Design review of the part built by this model. Coordinates are the model's own, in mm. A direction names the side the tool comes from. Round coordinates to 2 decimals unless told otherwise and drop trailing zeros. Write each loop counter-clockwise with the first axis right and the second up, starting at its lowest first coordinate (ties: lowest second). Pieces come first, ordered by that corner, then holes. Notation, with made-up numbers: M 3,-27.5 L 52,-27.5 A18 cw 52,-2.5 Z; hole C 77.25,-34.75 d9. An arc over 180 degrees is marked long. Use CSV: the item, a comma, the result in double quotes.
from build123d import *

# Parameters (mm, degrees)
BOSS_EXTRUDE1_DEPTH = 18
SKETCH2_R           = 5
BOSS_EXTRUDE2_DEPTH = 18.5
SKETCH3_W           = 10
SKETCH3_H           = 9.25
BOSS_EXTRUDE3_DEPTH = 35
DELETEFACE1_START   = 27.25
DELETEFACE1_DEPTH   = 9.25
SKETCH4_R           = 3
CUT_EXTRUDE1_DEPTH  = 124.902325662
SKETCH5_R           = 1
CUT_EXTRUDE4_DEPTH  = 123.576174145


# Read off the part's stored shape, not the designer's step: DeleteFace1
with BuildPart() as part:
    # Sketch1 → Boss-Extrude1 (new body)
    with BuildSketch(Plane(origin=(0, 0, 0), x_dir=(0, 1, 0), z_dir=(0, 0, 1))):
        with BuildLine():
            Line((-0.63860975, 30.836781145), (108.03933208, 17.892911363))
            ThreePointArc((108.03933208, 17.892911363), (115.421662674, 9.579146253), (108.03933208, 1.265381143))
            Line((108.03933208, 1.265381143), (-0.63860975, -11.678488639))
            ThreePointArc((-0.63860975, -11.678488639), (-24.578337326, 9.579146253), (-0.63860975, 30.836781145))
        make_face()
    extrude(amount=BOSS_EXTRUDE1_DEPTH)

    # Sketch2 → Boss-Extrude2 (add)
    with BuildSketch(Plane.XY.offset(18)):
        with Locations(Location((-9.579146253, -3.17045801, 0), (0, 0, 180))):
            Circle(SKETCH2_R)
    extrude(amount=BOSS_EXTRUDE2_DEPTH)

    # Sketch3 → Boss-Extrude3 (add)
    with BuildSketch(Plane(origin=(0, 0, 0), x_dir=(-1, 0, 0), z_dir=(0, 1, 0))):
        with Locations((9.579146253, 31.875)):
            Rectangle(SKETCH3_W, SKETCH3_H)
    extrude(amount=-BOSS_EXTRUDE3_DEPTH)

    # DeleteFace1 outline → DeleteFace1 (cut)
    with BuildSketch(Plane.XY.offset(DELETEFACE1_START)):
        with BuildLine():
            ThreePointArc((-5.712856558, 0), (-4.871097375, -1.486927267), (-4.579146253, -3.17045801))
            Line((-4.579146253, -3.17045801), (-4.579146253, 0))
            Line((-4.579146253, 0), (-5.712856558, 0))
        make_face()
        with BuildLine():
            Line((-14.579146253, 0), (-14.579146253, -3.17045801))
            ThreePointArc((-14.579146253, -3.17045801), (-14.287195131, -1.486927267), (-13.445435948, 0))
            Line((-13.445435948, 0), (-14.579146253, 0))
        make_face()
    extrude(amount=DELETEFACE1_DEPTH, mode=Mode.SUBTRACT)

    # Sketch4 → Cut-Extrude1 (cut, through all)
    with BuildSketch(Plane.YZ.offset(-4.579146253)):
        with Locations(Location((-28.17045801, 31.875, 0), (0, 0, 270))):
            Circle(SKETCH4_R)
    extrude(amount=-CUT_EXTRUDE1_DEPTH, mode=Mode.SUBTRACT)

    # Sketch5 → Cut-Extrude4 (cut, through all)
    with BuildSketch(Plane(origin=(0, 0, 27.25), x_dir=(1, 0, 0), z_dir=(0, 0, -1))):
        with Locations(Location((-10.579146253, 28.17045801, 0), (0, 0, 180))):
            Circle(SKETCH5_R)
    extrude(amount=-CUT_EXTRUDE4_DEPTH, mode=Mode.SUBTRACT)


solid = part.part
1) Add section A-A on z = 16.5. Write out the cut boundary in (x, y), then the cut area to 3 significant figures.
Answers:
outline,"M -30.84,-0.64 A21.41 ccw long 11.68,-0.64 L -1.27,108.04 A8.37 ccw -17.89,108.04 Z"
area,"4,140 mm²"
2) The part is to be moulded in two halves that separate along Z. For faces 3 (the face through (-4.579, -19, 32)), 4 (the face through (-10, -22, 27.25)), 5 (the face through (-10, -16, 36.5)), say which applies: released by +Z, released by -Z, zero draft, split by the parting line, or undercut.
Answers:
face 3,"zero draft"
face 4,"undercut"
face 5,"released by +Z"
3) Add section B-B on x = -16. Write out the cut boundary in (y, z).
Answers:
outline,"M -23.59,0 L 112.42,0 L 112.42,18 L -23.59,18 Z"
4) Add section C-C on z = 25. Write out the cut boundary in (x, y), then the cut area to 3 significant figures.
Answers:
outline,"C -9.58,-3.17 d10"
area,"78.5 mm²"
5) Machinability: for faces 1 (the face through (-9.75, 115.42, 8.87)), 2 (the face through (-14.579, -19, 32)), which of the approach directions +Z, -Z, +X, -X, +Y, -Y give a long, thin tool a straight path to every point of the face, cutting with its end or side? Answer none if there is none.
Answers:
face 1,"+Z, -Z, +Y"
face 2,"+Z, -X, +Y, -Y"
6) For pin 1 Ø13 at (x, y) = (-15, 33) entering from +Z; pin 2 Ø3 at (y, z) = (-17, 33.5) entering from +X; pin 3 Ø4.5 at (y, z) = (-22, 31) entering from -X; pin 4 Ø1.2 at (x, y) = (-10.58, -28.17) entering from +Z, all flat-tipped, find the tip position at first contact; note any pin that passes through.
Answers:
pin 1,"z = 18"
pin 2,"x = -4.58"
pin 3,"x = -14.58"
pin 4,"through"
7) Wall thickness on line 1 along Z through (x, y) = (6.5, 23); line 2 along X through (y, z) = (-4, 27.5); line 3 along Y through (x, z) = (-11, 30.5): over which ranges is each line inside the solid? List them lowest first. Write a range as [from, to].
Answers:
line 1,"[0, 18]"
line 2,"[-14.58, -4.58]"
line 3,"[-35, -30.84], [-25.5, 1.62]"
